Model file for the job. Use its own axes, mm. Give positions to 0.01 mm unless a question says otherwise; leave off trailing zeros. Order: outer loops, then holes, each group sorted by start corner. A loop starts at its lowest first (then second) coordinate and runs counter-clockwise, first axis right, second up. Notation, with made-up numbers: (54, -15.75) -> (106, -15.75) arc R21 ccw to (106, 22.25) -> close; hole circle Ø2 at (17.25, 37). An arc over 180 degrees is marked (long way). Answer in a Markdown table with one row per item. Add a question column.
from build123d import *

# Parameters (mm, degrees)
SKETCH1_R           = 47
SKETCH1_R_2         = 43
BOSS_EXTRUDE1_DEPTH = 1
CUT_EXTRUDE1_DEPTH  = 48


with BuildPart() as part:
    # Sketch1 → Boss-Extrude1 (new body, symmetric)
    with BuildSketch(Plane(origin=(0, 0, 0), x_dir=(1, 0, 0), z_dir=(0, 1, 0))):
        Circle(SKETCH1_R)
        Circle(SKETCH1_R_2, mode=Mode.SUBTRACT)
    extrude(amount=BOSS_EXTRUDE1_DEPTH, both=True)

    # Sketch2 → Cut-Extrude1 (cut, through all)
    with BuildSketch(Plane.XY):
        Polygon((-7.424621202, -6.717514421), (6.717514421, 7.424621202), (7.424621202, 6.717514421), (-6.717514421, -7.424621202), align=None)
    extrude(amount=-CUT_EXTRUDE1_DEPTH, mode=Mode.SUBTRACT)


solid = part.part
Item 1: Two-plate mould, pull along Y, no slides. Class faces 1 (the flat face through (-0.721, -0.014, -44.955)), 2 (the flat face through (21, -1, 38)), 3 (the flat face through (0.721, 0.014, -44.955)), 4 (the flat face through (21, 1, 38)): pulls with the +Y half, pulls with the -Y half, needs draft (parallel to the pull), parting line crosses it, or undercut.
Item 2: Saw through at A-A on z = 14. List the corners of the cut face in (x, y).
Item 3: Saw through at C-C on y = -0.55. List the corners of the cut face in (x, z), plus the area to 3 significant figures.
Item 4: Saw through at B-B on x = -21.5. List the corners of the cut face in (y, z).
Item 5: Wall check: line 1 (X direction, y = 0.3, z = 0); line 2 (Z direction, x = 0, y = 0.35); line 3 (Z direction, x = -8, y = -0.7). Give the ranges that are in metal, low to high.
Evaluation:
| question | item | result |
|---|---|---|
| 1 | face 1 | undercut |
| 1 | face 2 | pulls with the -Y half |
| 1 | face 3 | undercut |
| 1 | face 4 | pulls with the +Y half |
| 2 | outline | (-44.87, -1) -> (-40.66, -1) -> (-40.66, 1) -> (-44.87, 1) -> close; (40.66, -1) -> (44.87, -1) -> (44.87, 1) -> (40.66, 1) -> close |
| 3 | outline | (-1.26, -46.98) -> (-1.26, -42.98) arc R43 cw (long way) to (0.16, -43) -> (0.16, -47) arc R47 ccw (long way) to start |
| 3 | area | 1,130 mm2 |
| 4 | outline | (-1, -41.79) -> (1, -41.79) -> (1, -37.24) -> (-1, -37.24) -> close; (-1, 37.24) -> (1, 37.24) -> (1, 41.79) -> (-1, 41.79) -> close |
| 5 | line 1 | x = -47 to -43, 43 to 47 |
| 5 | line 2 | z = 43 to 47 |
| 5 | line 3 | z = -46.31 to -42.25, 42.25 to 46.31 |
